Geometry: see drawing. Coordinates: mm, zero at the bounding-box minimum. Give positions to 0.01 mm unless a question says otherwise; leave off trailing zeros. Loops run counter-clockwise (first coordinate to the right, second up) from the corner with the lowest first, then second, coordinate; pieces in that order, holes last. Notation, with made-up numbers: M 71,65 L 129,65 A25 ccw 129,99 Z; hole C 14.25,82 d9. An arc over 180 degrees is marked long. Put each result on its own line as item: value.
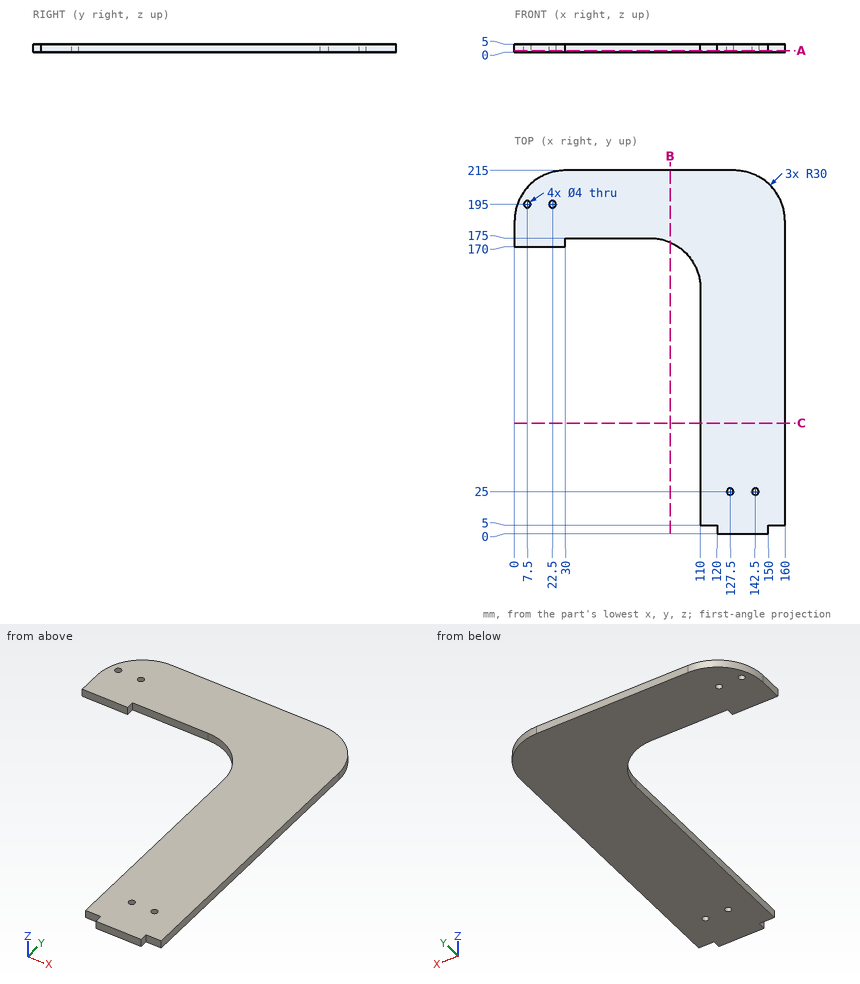
Item 1: Line query: probe 1 along Y at (x, z) = (127.5, 1.7); probe 2 along X at (y, z) = (195, 3.5); probe 3 along X at (y, z) = (24.5, 4.8). Output: solid intervals per line, ascending. Write a range as [from, to].
Output values:
probe 1: [0, 23], [27, 215]
probe 2: [1.72, 5.5], [9.5, 20.5], [24.5, 158.28]
probe 3: [110, 125.56], [129.44, 140.56], [144.44, 160]
Item 2: Pin query (flat end, axial travel): pin 1 Ø2.5 at (y, z) = (79.5, 1.5) entering from -X; pin 2 Ø1.5 at (x, z) = (10, 3.5) entering from -Y; pin 3 Ø12 at (x, y) = (101, 44.5) entering from +Z; pin 4 Ø2.5 at (x, z) = (117.5, 3.5) entering from -Y. Return the tip coordinate at first contact, or that it passes through.
Output values:
pin 1: x = 110
pin 2: y = 170
pin 3: through
pin 4: y = 5
Item 3: Section C-C on y = 65.5. Output: boundary loops of the cut face in (x, z), then the cut area to 3 significant figures.
Output values:
outline: M 110,0 L 160,0 L 160,5 L 110,5 Z
area: 250 mm²
Item 4: Section B-B on x = 92. Output: boundary loops of the cut face in (y, z).
Output values:
outline: M 172.5,0 L 215,0 L 215,5 L 172.5,5 Z
Item 5: Section A-A on z = 1.15. Output: boundary loops of the cut face in (x, y).
Output values:
outline: M 0,170 L 30,170 L 30,175 L 80,175 A30 cw 110,145 L 110,5 L 120,5 L 120,0 L 150,0 L 150,5 L 160,5 L 160,185 A30 ccw 130,215 L 30,215 A30 ccw 0,185 Z; hole C 7.5,195 d4; hole C 22.5,195 d4; hole C 127.5,25 d4; hole C 142.5,25 d4
